from build123d import *

# Parameters (mm, degrees)
SKETCH1_W               = 190.5
SKETCH1_H               = 254
BOSS_EXTRUDE1_DEPTH     = 6.35
SKETCH2_W               = 6.35
SKETCH2_H               = 12.7
CUT_EXTRUDE1_DEPTH      = 7.35
LPATTERN1_COUNT         = 9
LPATTERN1_PITCH         = 25.4
MIRROR1_COPY_1_SKETCH_W = 6.35
MIRROR1_COPY_1_SKETCH_H = 12.7
MIRROR1_COPY_1_DEPTH    = 7.35
MIRROR1_COPY_2_SKETCH_W = 6.35
MIRROR1_COPY_2_SKETCH_H = 12.7
MIRROR1_COPY_2_DEPTH    = 7.35
MIRROR1_COPY_3_SKETCH_W = 6.35
MIRROR1_COPY_3_SKETCH_H = 12.7
MIRROR1_COPY_3_DEPTH    = 7.35
MIRROR1_COPY_4_SKETCH_W = 6.35
MIRROR1_COPY_4_SKETCH_H = 12.7
MIRROR1_COPY_4_DEPTH    = 7.35
MIRROR1_COPY_5_SKETCH_W = 6.35
MIRROR1_COPY_5_SKETCH_H = 12.7
MIRROR1_COPY_5_DEPTH    = 7.35
MIRROR1_COPY_6_SKETCH_W = 6.35
MIRROR1_COPY_6_SKETCH_H = 12.7
MIRROR1_COPY_6_DEPTH    = 7.35
MIRROR1_COPY_7_SKETCH_W = 6.35
MIRROR1_COPY_7_SKETCH_H = 12.7
MIRROR1_COPY_7_DEPTH    = 7.35
MIRROR1_COPY_8_SKETCH_W = 6.35
MIRROR1_COPY_8_SKETCH_H = 12.7
MIRROR1_COPY_8_DEPTH    = 7.35
SKETCH3_W               = 12.7
SKETCH3_H               = 6.35
CUT_EXTRUDE2_DEPTH      = 7.35
LPATTERN2_COUNT         = 7
LPATTERN2_PITCH         = 25.4
MIRROR2_COPY_1_SKETCH_W = 12.7
MIRROR2_COPY_1_SKETCH_H = 6.35
MIRROR2_COPY_1_DEPTH    = 7.35
MIRROR2_COPY_2_SKETCH_W = 12.7
MIRROR2_COPY_2_SKETCH_H = 6.35
MIRROR2_COPY_2_DEPTH    = 7.35
MIRROR2_COPY_3_SKETCH_W = 12.7
MIRROR2_COPY_3_SKETCH_H = 6.35
MIRROR2_COPY_3_DEPTH    = 7.35
MIRROR2_COPY_4_SKETCH_W = 12.7
MIRROR2_COPY_4_SKETCH_H = 6.35
MIRROR2_COPY_4_DEPTH    = 7.35
MIRROR2_COPY_5_SKETCH_W = 12.7
MIRROR2_COPY_5_SKETCH_H = 6.35
MIRROR2_COPY_5_DEPTH    = 7.35
MIRROR2_COPY_6_SKETCH_W = 12.7
MIRROR2_COPY_6_SKETCH_H = 6.35
MIRROR2_COPY_6_DEPTH    = 7.35
SKETCH4_W               = 6.35
SKETCH4_H               = 25.4
CUT_EXTRUDE3_DEPTH      = 7.35


with BuildPart() as part:
    # Sketch1 → Boss-Extrude1 (new body)
    with BuildSketch(Plane(origin=(0, 0, 0), x_dir=(0, 0, -1), z_dir=(1, 0, 0))):
        Rectangle(SKETCH1_W, SKETCH1_H)
    extrude(amount=BOSS_EXTRUDE1_DEPTH)

    # Sketch2 → Cut-Extrude1 (cut, through all)
    with BuildSketch(Plane.ZY):
        with Locations((-92.075, -82.55)):
            Rectangle(SKETCH2_W, SKETCH2_H)
    cut_extrude1 = extrude(amount=-CUT_EXTRUDE1_DEPTH, mode=Mode.SUBTRACT)

    # LPattern1: Cut-Extrude1 ×9
    with Locations(*[(0, i * LPATTERN1_PITCH, 0) for i in range(1, LPATTERN1_COUNT)]):
        add(cut_extrude1, mode=Mode.SUBTRACT)

    # Mirror1: Cut-Extrude1 across plane
    add(cut_extrude1.mirror(Plane.XY), mode=Mode.SUBTRACT)

    # Mirror1 copy 1 sketch → Mirror1 copy 1 (cut, through all)
    with BuildSketch(Plane(origin=(0, 25.4, 0), x_dir=(0, 0, -1), z_dir=(-1, 0, 0))):
        with Locations((-92.075, 82.55)):
            Rectangle(MIRROR1_COPY_1_SKETCH_W, MIRROR1_COPY_1_SKETCH_H)
    extrude(amount=-MIRROR1_COPY_1_DEPTH, mode=Mode.SUBTRACT)

    # Mirror1 copy 2 sketch → Mirror1 copy 2 (cut, through all)
    with BuildSketch(Plane(origin=(0, 50.8, 0), x_dir=(0, 0, -1), z_dir=(-1, 0, 0))):
        with Locations((-92.075, 82.55)):
            Rectangle(MIRROR1_COPY_2_SKETCH_W, MIRROR1_COPY_2_SKETCH_H)
    extrude(amount=-MIRROR1_COPY_2_DEPTH, mode=Mode.SUBTRACT)

    # Mirror1 copy 3 sketch → Mirror1 copy 3 (cut, through all)
    with BuildSketch(Plane(origin=(0, 76.2, 0), x_dir=(0, 0, -1), z_dir=(-1, 0, 0))):
        with Locations((-92.075, 82.55)):
            Rectangle(MIRROR1_COPY_3_SKETCH_W, MIRROR1_COPY_3_SKETCH_H)
    extrude(amount=-MIRROR1_COPY_3_DEPTH, mode=Mode.SUBTRACT)

    # Mirror1 copy 4 sketch → Mirror1 copy 4 (cut, through all)
    with BuildSketch(Plane(origin=(0, 101.6, 0), x_dir=(0, 0, -1), z_dir=(-1, 0, 0))):
        with Locations((-92.075, 82.55)):
            Rectangle(MIRROR1_COPY_4_SKETCH_W, MIRROR1_COPY_4_SKETCH_H)
    extrude(amount=-MIRROR1_COPY_4_DEPTH, mode=Mode.SUBTRACT)

    # Mirror1 copy 5 sketch → Mirror1 copy 5 (cut, through all)
    with BuildSketch(Plane(origin=(0, 127, 0), x_dir=(0, 0, -1), z_dir=(-1, 0, 0))):
        with Locations((-92.075, 82.55)):
            Rectangle(MIRROR1_COPY_5_SKETCH_W, MIRROR1_COPY_5_SKETCH_H)
    extrude(amount=-MIRROR1_COPY_5_DEPTH, mode=Mode.SUBTRACT)

    # Mirror1 copy 6 sketch → Mirror1 copy 6 (cut, through all)
    with BuildSketch(Plane(origin=(0, 152.4, 0), x_dir=(0, 0, -1), z_dir=(-1, 0, 0))):
        with Locations((-92.075, 82.55)):
            Rectangle(MIRROR1_COPY_6_SKETCH_W, MIRROR1_COPY_6_SKETCH_H)
    extrude(amount=-MIRROR1_COPY_6_DEPTH, mode=Mode.SUBTRACT)

    # Mirror1 copy 7 sketch → Mirror1 copy 7 (cut, through all)
    with BuildSketch(Plane(origin=(0, 177.8, 0), x_dir=(0, 0, -1), z_dir=(-1, 0, 0))):
        with Locations((-92.075, 82.55)):
            Rectangle(MIRROR1_COPY_7_SKETCH_W, MIRROR1_COPY_7_SKETCH_H)
    extrude(amount=-MIRROR1_COPY_7_DEPTH, mode=Mode.SUBTRACT)

    # Mirror1 copy 8 sketch → Mirror1 copy 8 (cut, through all)
    with BuildSketch(Plane(origin=(0, 203.2, 0), x_dir=(0, 0, -1), z_dir=(-1, 0, 0))):
        with Locations((-92.075, 82.55)):
            Rectangle(MIRROR1_COPY_8_SKETCH_W, MIRROR1_COPY_8_SKETCH_H)
    extrude(amount=-MIRROR1_COPY_8_DEPTH, mode=Mode.SUBTRACT)

    # Sketch3 → Cut-Extrude2 (cut, through all)
    with BuildSketch(Plane.ZY):
        with Locations((-69.85, -123.825)):
            Rectangle(SKETCH3_W, SKETCH3_H)
    cut_extrude2 = extrude(amount=-CUT_EXTRUDE2_DEPTH, mode=Mode.SUBTRACT)

    # LPattern2: Cut-Extrude2 ×7
    with Locations(*[(0, 0, i * LPATTERN2_PITCH) for i in range(1, LPATTERN2_COUNT)]):
        add(cut_extrude2, mode=Mode.SUBTRACT)

    # Mirror2: Cut-Extrude2 across plane
    add(cut_extrude2.mirror(Plane.ZX), mode=Mode.SUBTRACT)

    # Mirror2 copy 1 sketch → Mirror2 copy 1 (cut, through all)
    with BuildSketch(Plane(origin=(0, 0, 25.4), x_dir=(0, 0, 1), z_dir=(-1, 0, 0))):
        with Locations((-69.85, 123.825)):
            Rectangle(MIRROR2_COPY_1_SKETCH_W, MIRROR2_COPY_1_SKETCH_H)
    extrude(amount=-MIRROR2_COPY_1_DEPTH, mode=Mode.SUBTRACT)

    # Mirror2 copy 2 sketch → Mirror2 copy 2 (cut, through all)
    with BuildSketch(Plane(origin=(0, 0, 50.8), x_dir=(0, 0, 1), z_dir=(-1, 0, 0))):
        with Locations((-69.85, 123.825)):
            Rectangle(MIRROR2_COPY_2_SKETCH_W, MIRROR2_COPY_2_SKETCH_H)
    extrude(amount=-MIRROR2_COPY_2_DEPTH, mode=Mode.SUBTRACT)

    # Mirror2 copy 3 sketch → Mirror2 copy 3 (cut, through all)
    with BuildSketch(Plane(origin=(0, 0, 76.2), x_dir=(0, 0, 1), z_dir=(-1, 0, 0))):
        with Locations((-69.85, 123.825)):
            Rectangle(MIRROR2_COPY_3_SKETCH_W, MIRROR2_COPY_3_SKETCH_H)
    extrude(amount=-MIRROR2_COPY_3_DEPTH, mode=Mode.SUBTRACT)

    # Mirror2 copy 4 sketch → Mirror2 copy 4 (cut, through all)
    with BuildSketch(Plane(origin=(0, 0, 101.6), x_dir=(0, 0, 1), z_dir=(-1, 0, 0))):
        with Locations((-69.85, 123.825)):
            Rectangle(MIRROR2_COPY_4_SKETCH_W, MIRROR2_COPY_4_SKETCH_H)
    extrude(amount=-MIRROR2_COPY_4_DEPTH, mode=Mode.SUBTRACT)

    # Mirror2 copy 5 sketch → Mirror2 copy 5 (cut, through all)
    with BuildSketch(Plane(origin=(0, 0, 127), x_dir=(0, 0, 1), z_dir=(-1, 0, 0))):
        with Locations((-69.85, 123.825)):
            Rectangle(MIRROR2_COPY_5_SKETCH_W, MIRROR2_COPY_5_SKETCH_H)
    extrude(amount=-MIRROR2_COPY_5_DEPTH, mode=Mode.SUBTRACT)

    # Mirror2 copy 6 sketch → Mirror2 copy 6 (cut, through all)
    with BuildSketch(Plane(origin=(0, 0, 152.4), x_dir=(0, 0, 1), z_dir=(-1, 0, 0))):
        with Locations((-69.85, 123.825)):
            Rectangle(MIRROR2_COPY_6_SKETCH_W, MIRROR2_COPY_6_SKETCH_H)
    extrude(amount=-MIRROR2_COPY_6_DEPTH, mode=Mode.SUBTRACT)

    # Sketch4 → Cut-Extrude3 (cut, through all)
    with BuildSketch(Plane.ZY):
        with Locations((-92.075, -114.3)):
            Rectangle(SKETCH4_W, SKETCH4_H)
    cut_extrude3 = extrude(amount=-CUT_EXTRUDE3_DEPTH, mode=Mode.SUBTRACT)

    # Mirror3: Cut-Extrude3 across plane
    add(cut_extrude3.mirror(Plane.XY), mode=Mode.SUBTRACT)


solid = part.part
Geometry: final body of the model. Coordinates: model frame, mm. A direction names the side the tool comes from. Give positions to 0.01 mm unless a question says otherwise; leave off trailing zeros. Write each loop counter-clockwise with the first axis right and the second up, starting at its lowest first coordinate (ties: lowest second). Pieces come first, ordered by that corner, then holes. Notation, with made-up numbers: M 48,47 L 80,47 A32 cw 80,78 Z; hole C -16,-29.75 d10. An arc over 180 degrees is marked long. Answer in a Markdown table with one row per item. Add a question column.
(1) Ray query, line 1 (Y direction, x = 3.25, z = 6.5); line 2 (Z direction, x = 4.75, y = -57.5). Return the intervals inside material, ascending.
(2) Section B-B on z = 7. Return loops of the section in (x, y).
(3) Reachability of faces 1 (the flat face through (3, -6, 88.9)), 2 (the flat face through (3, 25.4, -92)), 3 (the flat face through (3, -124, 25.4)), 4 (the flat face through (3, 124, 25.4)) from +Z, -Z, +X, -X, +Y, -Y: full face, straight path, thin tool, end or side. Return the list, or none.
(4) Mould query, pull axis Y, two halves, no side actions, for faces 5 (the flat face through (3, 124, 63.5)), 6 (the flat face through (3, 127, 19)), 7 (the flat face through (3, 76.2, -92)). Classes: +Y half, -Y half, draft (parallel to the pull), parting line (faces both ways), or undercut.
(5) Section A-A on y = -106. Return loops of the section in (x, z).
(6) First-contact query: pin 1 (1.9 mm diameter, centred on x = 4.5, z = 92, fed in from +Y); pin 2 (2 mm diameter, centred on x = 1.5, z = 9.5, fed in from +Y); pin 3 (3 mm diameter, centred on x = 4.5, z = -92.5, fed in from -Y). Flat tips, straight axial feed; report the tip coordinate or a pass-through.
Result set:
| question | item | result |
|---|---|---|
| 1 | line 1 | y = -120.65 to 120.65 |
| 1 | line 2 | z = -88.9 to 88.9 |
| 2 | outline | M 0,-120.65 L 6.35,-120.65 L 6.35,120.65 L 0,120.65 Z |
| 3 | face 1 | +Z, +X, -X |
| 3 | face 2 | -Z, +X, -X |
| 3 | face 3 | +X, -X, -Y |
| 3 | face 4 | +X, -X, +Y |
| 4 | face 5 | draft |
| 4 | face 6 | +Y half |
| 4 | face 7 | undercut |
| 5 | outline | M 0,-88.9 L 6.35,-88.9 L 6.35,88.9 L 0,88.9 Z |
| 6 | pin 1 | stops at y = 114.3 |
| 6 | pin 2 | stops at y = 120.65 |
| 6 | pin 3 | stops at y = -101.6 |
